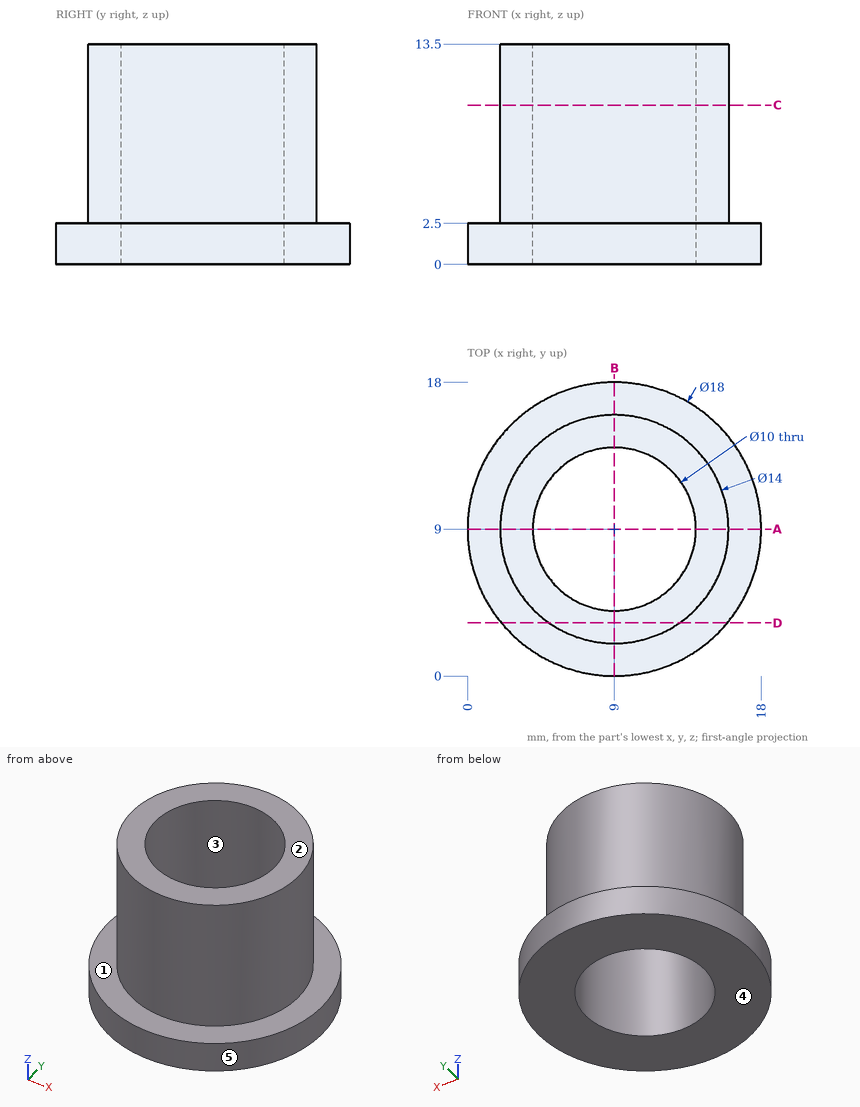
Here's the drawing with two shaded views (mm, measured from the low corner). I have some questions. A direction names the side the tool comes from. Round coordinates to 2 decimals unless told otherwise and drop trailing zeros. Write each loop counter-clockwise with the first axis right and the second up, starting at its lowest first coordinate (ties: lowest second). Pieces come first, ordered by that corner, then holes.
(1) Suppose I cut it at A-A on y = 9. Write out the boundary of the cut face in (x, z), and give its area (3 significant figures).
Findings below:
outline: (0, 0) - (4, 0) - (4, 13.5) - (2, 13.5) - (2, 2.5) - (0, 2.5) - close; (14, 0) - (18, 0) - (18, 2.5) - (16, 2.5) - (16, 13.5) - (14, 13.5) - close
area: 64.0 mm2
(2) Suppose I cut it at D-D on y = 3.25. Write out the boundary of the cut face in (x, z), and give its area (3 significant figures).
Findings below:
outline: (2.08, 0) - (15.92, 0) - (15.92, 2.5) - (12.99, 2.5) - (12.99, 13.5) - (5.01, 13.5) - (5.01, 2.5) - (2.08, 2.5) - close
area: 122 mm2
(3) Suppose I cut it at C-C on z = 9.75. Write out the boundary of the cut face in (x, y), and give its area (3 significant figures).
Findings below:
outline: circle Ø14 at (9, 9); hole circle Ø10 at (9, 9)
area: 75.4 mm2
(4) Thinking about a two-plate mould opening in Y: for the marked faces 3, 4 and 5, which applies, +Y half, -Y half, draft (parallel to the pull), parting line (faces both ways), or undercut?
Findings below:
face 3: undercut
face 4: draft
face 5: parting line
(5) Which directions (+Z, -Z, +X, -X, +Y, -Y) give clear straight access to the entire face, cutting with the end or side of a thin tool? Please do the marked faces 1 and 2.
Findings below:
face 1: +Z
face 2: +Z, +X, -X, +Y, -Y
(6) For pin 1 (3 mm diameter, centred on x = 11, z = 10, fed in from -Y); pin 2 (5 mm diameter, centred on y = 8.5, z = 10, fed in from -X); pin 3 (1 mm diameter, centred on y = 3, z = 4.5, fed in from -X), each with a flat end and sliding along its axis, tell me the tip position at first contact or that it passes through.
Findings below:
pin 1: stops at y = 2.02
pin 2: stops at x = 2
pin 3: stops at x = 4.67
(7) If I drill on probe 1 along Y at (x, z) = (9, 3.75); probe 2 along X at (y, z) = (8.75, 6.5); probe 3 along Z at (x, y) = (3.5, 3.5), over which ranges is the centre line in solid material (lowest first)?
Findings below:
probe 1: y = 2 to 4, 14 to 16
probe 2: x = 2 to 4.01, 13.99 to 16
probe 3: z = 0 to 2.5
